Design review of the part built by this model. Coordinates are the model's own, in mm. A direction names the side the tool comes from. Give positions to 0.01 mm unless a question says otherwise; leave off trailing zeros. Loops run counter-clockwise (first coordinate to the right, second up) from the corner with the lowest first, then second, coordinate; pieces in that order, holes last. Notation, with made-up numbers: M -18.75,-13.75 L -8.75,-13.75 A24 cw -8.75,19.25 Z; hole C 49.5,-19.5 d9. An arc over 180 degrees is marked long. Use a Markdown table: item, result. Add a question column.
(1) Add section C-C, the plane z = 0. State how many separate pieces and enclosed holes the cut face has, then the cut area to 3 significant figures.
(2) For probe 1 along Z at (x, y) = (-37, -4); probe 2 along Y at (x, z) = (-23.5, 3); probe 3 along X at (y, z) = (-39, -7), list the stretches that pass through material, from the lowest coordinate up.
(3) For faces 1 (the face through (19.05, -36, 0)), 2 (the face through (-43.109, 39.876, 0.643)), 3 (the face through (-27.1, 22, -4)), 4 (the face through (34, -59.232, 0)), list the 3-axis set-ups (+Z, -Z, +X, -X, +Y, -Y) from which the entire face can be reached by the end or side of a thin tool; tool diameter is ignored.
(4) Draft analysis for pull direction Z (two halves, no side actions). For faces 5 (the face through (0, -21.132, 0)), 6 (the face through (-30.32, 20.457, 0.451)), 7 (the face through (-2, -8, 25.4)), state which applies: pulls with the +Z half, pulls with the -Z half, needs draft (parallel to the pull), parting line crosses it, or undercut.
(5) Insertion check: pin 1 Ø5 at (y, z) = (24, -4) entering from -X; pin 2 Ø11 at (y, z) = (-41.5, -0.5) entering from +X; pin 3 Ø2.5 at (y, z) = (33.94, 0) entering from +X; pin 4 Ø15.5 at (y, z) = (-44.23, 0) entering from -X. Each pin has a flat end and moves straight along its axis. Give the tip position at first contact, or say it passes through.
(6) Add section D-D, the plane x = 35. Give the boundary of the cut face in (y, z).
(7) Add section A-A, the plane x = 0.5. Give the boundary of the cut face in (y, z), then the cut area to 3 significant figures.
(8) Add section B-B, the plane y = -43. Give the boundary of the cut face in (x, z), then the cut area to 3 significant figures.
```python
from build123d import *

# Parameters (mm, degrees)
F0_W      = 101.6
F0_H      = 101.6
F1_DEPTH  = 25.4
F2_R      = 18
F3_DEPTH  = 76.2
F4_R      = 18
F5_DEPTH  = 19.05
F6_R      = 1.5
F7_DEPTH  = 25
F8_R      = 11
F9_DEPTH  = 25.4
F10_R     = 11
F11_DEPTH = 25.4
F12_W     = 38.1
F12_H     = 43.3616997044
F13_DEPTH = 50.801
F14_R     = 6
F15_DEPTH = 76.201
F17_DEPTH = 19.05


# Not quite as in the source:
# - a length typed as a fraction of an inch, garbled in the dataset ("3 / 203.2 mm" for 3/8 in), is restored


with BuildPart() as f1:
    # F0 (on Top) → F1 (new body, symmetric)
    with BuildSketch(Plane.XY):
        with Locations((-1.7001610249, -8.4323180143)):
            Rectangle(F0_W, F0_H)
    extrude(amount=F1_DEPTH, both=True)

    # F2 (on face) → F3 (cut)
    with BuildSketch(Plane.YZ.offset(49.0998389751)):
        with Locations((21.8872688711, 0)):
            Circle(F2_R)
    extrude(amount=-F3_DEPTH, mode=Mode.SUBTRACT)

    # F4 (on face) → F5 (cut)
    with BuildSketch(Plane(origin=(-52.5001610249, 0, 0), x_dir=(0, -1, 0), z_dir=(-1, 0, 0))):
        with Locations((-21.8872688711, 0)):
            Circle(F4_R)
    extrude(amount=-F5_DEPTH, mode=Mode.SUBTRACT)

    # F6 (on face) → F7 (cut)
    with BuildSketch(Plane(origin=(-33.4501610249, 0, 0), x_dir=(0, -1, 0), z_dir=(-1, 0, 0))):
        with Locations((-21.8872688711, 0)):
            Circle(F6_R)
        with Locations((-9.838248603, 0)):
            Circle(F6_R)
        with Locations((-15.8627587371, 10.4347576428)):
            Circle(F6_R)
        with Locations((-27.9117790051, 10.4347576428)):
            Circle(F6_R)
        with Locations((-33.9362891391, 0)):
            Circle(F6_R)
        with Locations((-27.9117790051, -10.4347576428)):
            Circle(F6_R)
        with Locations((-15.8627587371, -10.4347576428)):
            Circle(F6_R)
    extrude(amount=-F7_DEPTH, mode=Mode.SUBTRACT)

    # F8 (on face) → F9 (cut)
    with BuildSketch(Plane(origin=(-52.5001610249, 0, 0), x_dir=(0, -1, 0), z_dir=(-1, 0, 0))):
        with Locations((44.2323180143, 0)):
            Circle(F8_R)
    extrude(amount=-F9_DEPTH, mode=Mode.SUBTRACT)

    # F10 (on face) → F11 (cut)
    with BuildSketch(Plane.YZ.offset(49.0998389751)):
        with Locations((-44.2323180143, 0)):
            Circle(F10_R)
    extrude(amount=-F11_DEPTH, mode=Mode.SUBTRACT)

    # F12 (on face) → F13 (cut, through all)
    with BuildSketch(Plane(origin=(0, 0, -25.4), x_dir=(1, 0, 0), z_dir=(0, 0, -1))):
        with Locations((0, 42.8131678666)):
            Rectangle(F12_W, F12_H)
    extrude(amount=-F13_DEPTH, mode=Mode.SUBTRACT)

    # F14 (on face) → F15 (cut, through all)
    with BuildSketch(Plane(origin=(-27.1001610249, 0, 0), x_dir=(0, -1, 0), z_dir=(-1, 0, 0))):
        with Locations((44.2323180143, 0)):
            Circle(F14_R)
    extrude(amount=-F15_DEPTH, mode=Mode.SUBTRACT)

    # F16 (on face) → F17 (cut)
    with BuildSketch(Plane(origin=(-52.5001610249, 0, 0), x_dir=(0, -1, 0), z_dir=(-1, 0, 0))):
        with BuildLine():
            Line((-21.8872688711, -10), (44.2323180143, -10))
            ThreePointArc((44.2323180143, -10), (54.2323180143, 0), (44.2323180143, 10))
            Line((44.2323180143, 10), (-21.8872688711, 10))
            ThreePointArc((-21.8872688711, 10), (-31.8872688711, 0), (-21.8872688711, -10))
        make_face()
    extrude(amount=-F17_DEPTH, mode=Mode.SUBTRACT)


solid = f1.part
```
Established:
| question | item | result |
|---|---|---|
| 1 | separate pieces | 6 |
| 1 | enclosed holes | 0 |
| 1 | area | 3,410 mm^2 |
| 2 | probe 1 | -25.4 to -10, 10 to 25.4 |
| 2 | probe 2 | -59.23 to -49.43, -39.04 to 4.14, 39.64 to 42.37 |
| 2 | probe 3 | -27.1 to -19.05, 19.05 to 23.7 |
| 3 | face 1 | +Z, -Z, -Y |
| 3 | face 2 | -X |
| 3 | face 3 | +X |
| 3 | face 4 | +Z, -Z, +X, -X, -Y |
| 4 | face 5 | needs draft |
| 4 | face 6 | undercut |
| 4 | face 7 | pulls with the +Z half |
| 5 | pin 1 | x = -33.45 |
| 5 | pin 2 | x = 23.7 |
| 5 | pin 3 | through |
| 5 | pin 4 | x = -27.1 |
| 6 | outline | M -59.23,-25.4 L 42.37,-25.4 L 42.37,25.4 L -59.23,25.4 Z; hole C -44.23,0 d22; hole C 21.89,0 d36 |
| 7 | outline | M -21.13,-25.4 L 42.37,-25.4 L 42.37,25.4 L -21.13,25.4 Z; hole C 21.89,0 d36 |
| 7 | area | 2,210 mm^2 |
| 8 | outline | M -52.5,-25.4 L -19.05,-25.4 L -19.05,-5.87 L -27.1,-5.87 L -27.1,-10.93 L -52.5,-10.93 Z; M -52.5,10.93 L -27.1,10.93 L -27.1,5.87 L -19.05,5.87 L -19.05,25.4 L -52.5,25.4 Z; M 19.05,-25.4 L 49.1,-25.4 L 49.1,-10.93 L 23.7,-10.93 L 23.7,-5.87 L 19.05,-5.87 Z; M 19.05,5.87 L 23.7,5.87 L 23.7,10.93 L 49.1,10.93 L 49.1,25.4 L 19.05,25.4 Z |
| 8 | area | 1,970 mm^2 |
